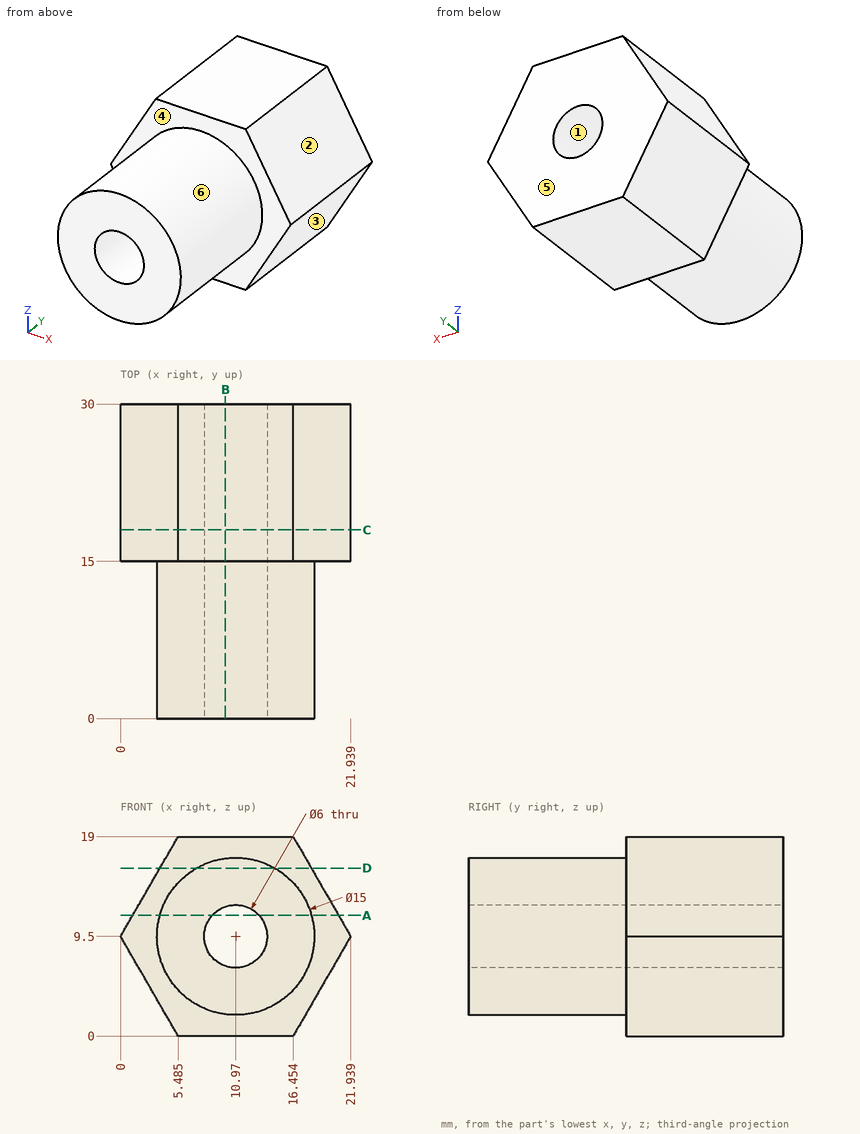
Source: three-view drawing plus pictorial views. Frame: mm from the lowest corner of the part. A direction names the side the tool comes from. Give positions to 0.01 mm unless a question says otherwise; leave off trailing zeros. Write each loop counter-clockwise with the first axis right and the second up, starting at its lowest first coordinate (ties: lowest second). Pieces come first, ordered by that corner, then holes.
(1) Cut plane A-A, the plane z = 11.5. Return loops of the section in (x, y) (1 decimal), then the cut area to 3 significant figures.
(2) Cut plane C-C, the plane y = 18. Return loops of the section in (x, z) (1 decimal), then the cut area to 3 significant figures.
(3) Cut plane B-B, the plane x = 10. Return loops of the section in (y, z).
(4) Ray query, line 1 (X direction, y = 12.5, z = 9.5); line 2 (Y direction, x = 4, z = 6.5); line 3 (X direction, y = 3, z = 14.75) (1 decimal). Return the intervals inside material, ascending.
(5) Cut plane D-D, the plane z = 16. Return loops of the section in (x, y), then the cut area to 3 significant figures.
(6) Access query for the marked faces 5 and 6. Directions: +Z, -Z, +X, -X, +Y, -Y. A direction counts if a zero-diameter tool reaches every point of the face in a straight line with its end or side. Return the directions, or none.
(7) First-contact query: P1, Ø12, axis at x = 14, y = 7.5, coming from the +Z side; P2, Ø2, axis at y = 8.5, z = 12.5, coming from the -X side. Flat tips, straight axial feed; report the tip coordinate or a pass-through.
(8) Mould query, pull axis Z, two halves, no side actions, for the marked faces 1, 2, 3 and 4. Classes: released by +Z, released by -Z, zero draft, split by the parting line, or undercut.
Values follow:
1. outline: (1.2, 15) - (3.7, 15) - (3.7, 0) - (8.7, 0) - (8.7, 30) - (1.2, 30) - close; (13.2, 0) - (18.2, 0) - (18.2, 15) - (20.8, 15) - (20.8, 30) - (13.2, 30) - close
1. area: 377 mm2
2. outline: (0, 9.5) - (5.5, 0) - (16.5, 0) - (21.9, 9.5) - (16.5, 19) - (5.5, 19) - close; hole circle Ø6 at (11, 9.5)
2. area: 284 mm2
3. outline: (0, 2.06) - (15, 2.06) - (15, 0) - (30, 0) - (30, 6.66) - (0, 6.66) - close; (0, 12.34) - (30, 12.34) - (30, 19) - (15, 19) - (15, 16.94) - (0, 16.94) - close
4. line 1: x = 3.47 to 7.97, 13.97 to 18.47
4. line 2: y = 15 to 30
4. line 3: x = 5.6 to 16.3
5. outline: (3.75, 15) - (7.23, 15) - (7.23, 0) - (14.71, 0) - (14.71, 15) - (18.19, 15) - (18.19, 30) - (3.75, 30) - close
5. area: 329 mm2
6. face 5: +Z, -Z, +X, -X, +Y
6. face 6: -Y
7. P1: stops at z = 17
7. P2: stops at x = 3.74
8. face 1: undercut
8. face 2: released by +Z
8. face 3: released by -Z
8. face 4: zero draft
